Autodesk Inventor part; units mm, degrees
ref_plane "Work Plane1" through (-20, 125, -125) normal (0, 1, 0) x (-1, 0, 0)
ref_plane "YZ Plane" through (0, 0, 0) normal (1, 0, 0) x (0, 1, 0)
ref_plane "XY Plane" through (0, 0, 0) normal (0, 0, 1) x (1, 0, 0)
sketch "Sketch1" plane through (0, 0, 0) normal (1, 0, 0) x (0, 1, 0)
  line L0 (0, 175) -> (0, -175) construction
  line L1 (-175, 0) -> (175, 0) construction
  line L2 (125, 125) -> (-125, 125)
  line L3 (-125, 125) -> (-125, -125)
  line L4 (-125, -125) -> (125, -125)
  line L5 (125, -125) -> (125, 125)
  point P0 (0, 0)
  dimension "d0" = 250
  dimension "d1" = 250
extrude "Main_Body" add sketch "Sketch1" along normal mid plane 40
sketch "Sketch4" plane through (-20, 0, 0) normal (-1, 0, 0) x (0, 0, 1)
  line L0 (-175, 0) -> (175, 0) construction
  line L1 (0, 175) -> (0, -175) construction
  line L2 (-55, 100) -> (-25, 100) construction
  line L3 (-55, -100) -> (-25, -100) construction
  line L4 (-40, 100) -> (-40, -100) construction
  line L5 (20, 10) -> (97.4597, -10) construction
  point P0 (0, 0)
  dimension "d10" = 30
  dimension "d12" = 40
  dimension "d13" = 200
  dimension "d21" = 80
  dimension "d22" = 60
  dimension "d23" = 10
  dimension "d24" = 10
hole "Hole1" at (-20, 100, -55) at (-20, 100, -25) at (-20, -100, -55) at (-20, -100, -25) at (-20, 10, 20) at (-20, -10, 97.4597) direction (1, 0, 0) diameter 6 end through all
sketch "Sketch5" plane through (-20, 0, 0) normal (-1, 0, 0) x (0, 0, 1)
  line L0 (125, 125) -> (-125, 125)
  line L1 (-75, 125) -> (-75, 85)
  line L2 (-75, 85) -> (-5, 85)
  line L3 (-5, 85) -> (-5, 125)
  line L4 (-40, 100) -> (-40, -100) construction
  line L5 (-175, 0) -> (175, 0) construction
  line L6 (-75, -125) -> (-75, -85)
  line L7 (-75, -85) -> (-5, -85)
  line L8 (-5, -85) -> (-5, -125)
  line L9 (-125, -125) -> (125, -125)
  circle A0 centre (-55, 100) radius 3
  circle A1 centre (-25, 100) radius 3
  circle A2 centre (-55, -100) radius 3
  circle A3 centre (-25, -100) radius 3
  point P0 (0, 0)
  dimension "d32" = 40
  dimension "d33" = 70
extrude "L: Rock End Bracket Pocket" cut sketch "Sketch5" against normal up to surface (20 mm away)
sketch "Sketch8" plane through (20, 0, 0) normal (1, 0, 0) x (0, 0, -1)
  line L0 (40, 100) -> (40, -100) construction
  line L1 (-125, 125) -> (125, 125)
  line L2 (9.0545, 125) -> (9.0545, 85.102)
  line L3 (9.0545, 85.102) -> (70.9455, 85.102)
  line L4 (70.9455, 85.102) -> (70.9455, 125)
  line L5 (-175, 0) -> (175, 0) construction
  line L6 (9.0545, -125) -> (9.0545, -85.102)
  line L7 (9.0545, -85.102) -> (70.9455, -85.102)
  line L8 (70.9455, -85.102) -> (70.9455, -125)
  line L9 (-125, -125) -> (125, -125)
  circle A0 centre (25, 100) radius 3
  circle A1 centre (55, 100) radius 3
  circle A2 centre (25, -100) radius 3
  circle A3 centre (55, -100) radius 3
  point P0 (0, 0)
  dimension "d48" = 61.891
  dimension "d49" = 39.898
extrude "R: Rod End Bracket Pocket" [suppressed]
sketch "Sketch9" plane through (-20, 0, 0) normal (-1, 0, 0) x (0, 0, 1)
  line L0 (-40, 100) -> (-40, -100) construction
  line L1 (-175, 0) -> (175, 0) construction
  circle A0 centre (-40, 0) radius 28.5745
  point P0 (0, 0)
  dimension "d52" = 57.149
extrude "Axle Bore" [suppressed]
sketch "Sketch10" plane through (-20, 0, 0) normal (-1, 0, 0) x (0, 0, 1)
  circle A0 centre (-40, 0) radius 27.5
  circle A1 centre (-40, 0) radius 37.9265
  point P0 (0, 0)
  dimension "d55" = 75.853
extrude "Bearing Pocket 1" [suppressed]
sketch "Sketch11" plane through (20, 0, 0) normal (1, 0, 0) x (0, 0, -1)
  circle A0 centre (40, 0) radius 27.5
  circle A1 centre (40, 0) radius 38.383
  point P0 (0, 0)
  dimension "d58" = 76.766
extrude "Bearing Pocket 2" [suppressed]
ref_plane "Work Plane1" through (-20, 125, -125) normal (0, 1, 0) x (-1, 0, 0)
sketch "Sketch12" plane through (-20, 125, -125) normal (0, 1, 0) x (-1, 0, 0)
  line L0 (-20, -50) -> (-20, 300) construction
  line L1 (-48, 125) -> (8, 125) construction
  point P0 (-20, 125)
  point P1 (0, 85)
  point P2 (0, 85)
  point P3 (0, 85)
  point P4 (-20, 20.88)
  dimension "d61" = 64.12
hole "Hole4" [suppressed]
sketch "Sketch13" plane through (20, 125, -125) normal (0, 0, -1) x (-1, 0, 0)
  line L0 (20, -300) -> (20, 50) construction
  line L1 (-8, -125) -> (48, -125) construction
  line L2 (40, -203.192) -> (0, -203.192)
  line L3 (0, -203.192) -> (0, -230.998)
  line L4 (0, -230.998) -> (40, -230.998)
  line L5 (40, -230.998) -> (40, -203.192)
  line L6 (0, -217.095) -> (40, -217.095) construction
  line L7 (0, -250) -> (0, 0)
  line L8 (40, 0) -> (40, -250)
  point P0 (20, -125)
  dimension "d69" = 92.095
  dimension "d70" = 27.806
extrude "Extrusion9" [suppressed]
equation "\"d32\" = Rod_End_Bracket_Slot_Height"
equation "\"d33\" = Rod_End_Bracket_Slot_Width"
equation "\"Rod_End_Bracket_Slot_Height\" = 40"
equation "\"Rod_End_Bracket_Slot_Width\" = 70"
properties part number "Suspension_Upright_V2_Topology_Baseline_V1"
CAD build for the part. Positions are in the model's coordinates, mm. A direction names the side the tool comes from. Coordinates: 2 decimals unless noted, no trailing zeros. Loops run counter-clockwise (first coordinate to the right, second up) from the corner with the lowest first, then second, coordinate; pieces in that order, holes last. Notation, with made-up numbers: (-37, 46) - (-6, 46) arc R19 cw to (-6, 82) - close; hole circle Ø4 at (-37, -13). An arc over 180 degrees is marked (long way). Write item = value, one per line. Start each with the question number.
Q1. Flat gauge pins, fed straight in: pin 1 Ø6 at (x, z) = (-13, -47.5) entering from +Y; pin 2 Ø7 at (y, z) = (-100, -55) entering from -X; pin 3 Ø3.5 at (y, z) = (-10, 97.46) entering from -X; pin 4 Ø7 at (y, z) = (10, 20) entering from +X. Where does each tip first touch, or does it go through?
Q2. Which spindle directions (+Z, -Z, +X, -X, +Y, -Y) get a long thin tool onto all of the face, cutting with end or side? Do faces 1 (the flat face through (-10, 105, -75)), 2 (the flat face through (-10, -105, -75)), 3 (the cylindrical face through (10.14, -97.07, -25.65)). Say none if no direction does.
Q3. Cut at A-A, the plane z = -25. List the corners of the cut face in (x, y).
Q4. Drill centre lines: L1, parallel to Y at x = 13, z = -55; L2, parallel to Z at x = 12, y = -100; L3, parallel to Z at x = -16.5, y = -92. Where is each one in solid material? Low to high.
Q5. Cut at B-B, the plane y = 100. List the corners of the cut face in (x, z).
Q6. Pull direction Z, two halves, no side cores. Call faces 4 (the flat face through (0, -105, -40)), 5 (the flat face through (-10, -105, -5)), 6 (the flat face through (0, -125, 2)), 7 (the flat face through (0, 2, 125)): pulls with the +Z half, pulls with the -Z half, needs draft (parallel to the pull), parting line crosses it, or undercut.
Computed:
q1.pin_1 = 85
q1.pin_2 = 0
q1.pin_3 = through
q1.pin_4 = 20
q2.face_1 = -X, +Y
q2.face_2 = -X, -Y
q2.face_3 = +X, -X
q3.outline = (-20, -85) - (0, -85) - (0, -97) - (20, -97) - (20, 97) - (0, 97) - (0, 85) - (-20, 85) - close; (0, -125) - (20, -125) - (20, -103) - (0, -103) - close; (0, 103) - (20, 103) - (20, 125) - (0, 125) - close
q4.L1 = -125 to -103, -97 to 97, 103 to 125
q4.L2 = -125 to -58, -52 to -28, -22 to 125
q4.L3 = -125 to -75, -5 to 125
q5.outline = (-20, -125) - (20, -125) - (20, -58) - (0, -58) - (0, -75) - (-20, -75) - close; (-20, -5) - (0, -5) - (0, -22) - (20, -22) - (20, 125) - (-20, 125) - close; (0, -52) - (20, -52) - (20, -28) - (0, -28) - close
q6.face_4 = undercut
q6.face_5 = undercut
q6.face_6 = needs draft
q6.face_7 = pulls with the +Z half
